Design review of the part built by this model. Coordinates are the model's own, in mm. Face numbers are marked on the shaded views. A direction names the side the tool comes from. Round coordinates to 2 decimals unless told otherwise and drop trailing zeros. Write each loop counter-clockwise with the first axis right and the second up, starting at its lowest first coordinate (ties: lowest second). Pieces come first, ordered by that corner, then holes. Notation, with made-up numbers: M 66,43 L 70,43 A17 cw 70,55 Z; hole C -8.75,61.5 d5. An arc over 180 degrees is marked long. One line per question, with ' | ' between items. Start each with the question number.
Item 1: Draft analysis for pull direction X (two halves, no side actions). For the marked faces 1, 2 and 3, state which applies: released by +X, released by -X, zero draft, split by the parting line, or undercut.
Item 2: Add section B-B, the plane z = 14. State the section outline as (x, y) points, and give its area (3 significant figures).
Item 3: For L1, parallel to Z at x = -85.5, y = -1; L2, parallel to Z at x = -15, y = -28.5; L3, parallel to X at y = 14, z = 60.5, list the stretches that pass through material, from the lowest coordinate up.
Item 4: Insertion check: pin 1 Ø4 at (x, y) = (-70.5, 32.5) entering from -Z; pin 2 Ø5 at (x, z) = (-53.5, 36) entering from -Y; pin 3 Ø0.8 at (y, z) = (3, 1) entering from +X; pin 4 Ø0.9 at (y, z) = (-20.5, 1) entering from +X. Each pin has a flat end and moves straight along its axis. Give the tip position at first contact, or say it passes through.
Item 5: Machinability: for the marked faces 4, 5, 6 and 7, which of the approach directions +Z, -Z, +X, -X, +Y, -Y give a long, thin tool a straight path to every point of the face, cutting with its end or side? Answer none if there is none.
Item 6: Add section A-A, the plane z = 52. State the section outline as (x, y) points, and give its area (3 significant figures).
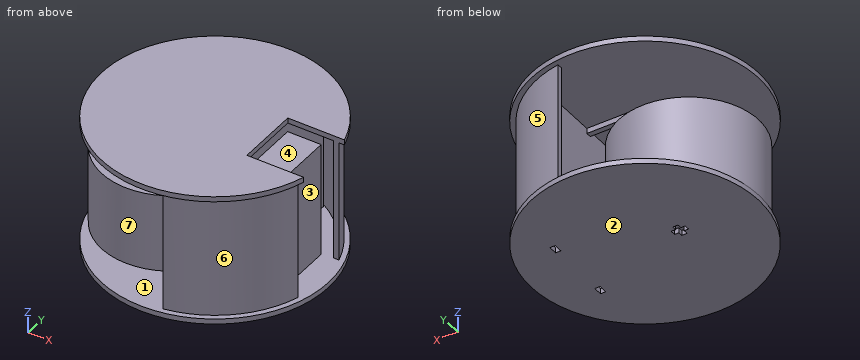
```python
from build123d import *

# Parameters (mm, degrees)
F0_W      = 19.2
F0_H      = 34.5
F1_DEPTH  = 68.5
F2_R      = 65
F2_W      = 3
F2_H      = 5
F3_DEPTH  = 3
F4_R      = 40
F5_DEPTH  = 45
F6_W      = 3
F6_H      = 36
F6_H_2    = 32.1239784062
F7_DEPTH  = 70
F11_DEPTH = 3
F13_DEPTH = 3


# Not quite as in the source:
# - a feature names something its author has since deleted; it is built from what else it names
# - the program builds the solid bodies; features that only make, move or delete a surface that nothing else refers to are left out


with BuildPart() as f1:
    # F0 (on Top) → F1 (new body)
    with BuildSketch(Plane.XY):
        Rectangle(F0_W, F0_H)
    extrude(amount=F1_DEPTH)

    # F2 (on Top) → F3 (join)
    with BuildSketch(Plane.XY):
        with Locations((-40, 0)):
            Circle(F2_R)
        with Locations((-13.5, -12.5)):
            Rectangle(F2_W, F2_H, mode=Mode.SUBTRACT)
        with Locations((-1.5, -19.75)):
            Rectangle(F2_W, F2_H, mode=Mode.SUBTRACT)
        Polygon((-58.5, -4), (-61.5, -4), (-61.5, -1.5), (-64, -1.5), (-64, 1.5), (-61.5, 1.5), (-61.5, 4), (-58.5, 4), (-58.5, 1.5), (-56, 1.5), (-56, -1.5), (-58.5, -1.5), align=None, mode=Mode.SUBTRACT)
        with Locations((-1.5, 19.75)):
            Rectangle(F2_W, F2_H, mode=Mode.SUBTRACT)
        with Locations((-13.5, -12.5)):
            Rectangle(F2_W, F2_H)
    extrude(amount=F3_DEPTH)

    # F4 (on face) → F5 (join)
    with BuildSketch(Plane.XY.offset(3)):
        with Locations((-65, 0)):
            Circle(F4_R)
    extrude(amount=F5_DEPTH)

    # F6 (on face) → F7 (join)
    with BuildSketch(Plane.XY.offset(3)):
        with Locations((-12, 0)):
            Rectangle(F6_W, F6_H)
        with Locations((-12, 34.0619892031)):
            Rectangle(F6_W, F6_H_2)
        with Locations((-12, -34.0619892031)):
            Rectangle(F6_W, F6_H_2)
        with BuildLine():
            Line((19.3295878968, -18), (16.1871871515, -18))
            ThreePointArc((16.1871871515, -18), (-1.2944625099, -44.5295561128), (-30, -58.1463670404))
            Line((-30, -58.1463670404), (-30, -61.1882341631))
            ThreePointArc((-30, -61.1882341631), (0.8405904954, -46.6481100151), (19.3295878968, -18))
        make_face()
        with BuildLine():
            Line((-30, 61.1882341631), (-30, 58.1463670404))
            ThreePointArc((-30, 58.1463670404), (-1.2944625099, 44.5295561128), (16.1871871515, 18))
            Line((16.1871871515, 18), (19.3295878968, 18))
            ThreePointArc((19.3295878968, 18), (0.8405904954, 46.6481100151), (-30, 61.1882341631))
        make_face()
    extrude(amount=F7_DEPTH)

    # F10 (on offset) → F11 (join)
    with BuildSketch(Plane.XY.offset(73)):
        with BuildLine():
            ThreePointArc((22.4579858785, 18), (-105, 0), (22.4579858785, -18))
            Line((22.4579858785, -18), (-10, -18))
            Line((-10, -18), (-10, 18))
            Line((-10, 18), (22.4579858785, 18))
        make_face()
    extrude(amount=F11_DEPTH)

    # F12 (on face) → F13 (join)
    with BuildSketch(Plane(origin=(0, 0, 73), x_dir=(1, 0, 0), z_dir=(0, 0, -1))):
        with BuildLine():
            Line((-13.5, -10.5), (-13.5, -7.5))
            Line((-13.5, -7.5), (-40, -7.5))
            ThreePointArc((-40, -7.5), (-47.5, 0), (-40, 7.5))
            Line((-40, 7.5), (-13.5, 7.5))
            Line((-13.5, 7.5), (-13.5, 10.5))
            Line((-13.5, 10.5), (-40, 10.5))
            ThreePointArc((-40, 10.5), (-50.5, 0), (-40, -10.5))
            Line((-40, -10.5), (-13.5, -10.5))
        make_face()
    extrude(amount=F13_DEPTH)


solid = f1.part
```
Computed values:
1) face 1: undercut | face 2: zero draft | face 3: released by +X
2) outline: C -65,0 d80; M -30,-61.19 A62 ccw 19.33,-18 L 16.19,-18 A59 cw -30,-58.15 Z; M -30,58.15 A59 cw 16.19,18 L 19.33,18 A62 ccw -30,61.19 Z; M -13.5,-50.12 L -10.5,-50.12 L -10.5,50.12 L -13.5,50.12 Z; M -9.6,-17.25 L 9.6,-17.25 L 9.6,17.25 L -9.6,17.25 Z | area: 6,390 mm^2
3) L1: z = 0 to 48, 73 to 76 | L2: z = 0 to 3, 73 to 76 | L3: x = -13.5 to -10.5, -9.6 to 9.6
4) pin 1: stops at z = 0 | pin 2: stops at y = -38.97 | pin 3: stops at x = 24.95 | pin 4: stops at x = 21.83
5) face 4: +Z, +X | face 5: +X, +Y | face 6: +X, -Y | face 7: none
6) outline: M -30,-61.19 A62 ccw 19.33,-18 L 16.19,-18 A59 cw -30,-58.15 Z; M -30,58.15 A59 cw 16.19,18 L 19.33,18 A62 ccw -30,61.19 Z; M -13.5,-50.12 L -10.5,-50.12 L -10.5,50.12 L -13.5,50.12 Z; M -9.6,-17.25 L 9.6,-17.25 L 9.6,17.25 L -9.6,17.25 Z | area: 1,360 mm^2
